from build123d import *

# Parameters (mm, degrees)
BOSS_EXTRUDE2_DEPTH = 230
SKETCH2_R           = 3
CUT_EXTRUDE1_DEPTH  = 4
SKETCH3_R           = 1.55
CUT_EXTRUDE2_DEPTH  = 4
LPATTERN1_COUNT     = 12
LPATTERN1_PITCH     = 20
SKETCH4_W           = 103
SKETCH4_H           = 312
SKETCH4_R           = 11.05
SKETCH4_R_2         = 1.55
SKETCH4_W_2         = 10
SKETCH4_H_2         = 12
BOSS_EXTRUDE3_DEPTH = 4.75
SKETCH5_R           = 1.25
CUT_EXTRUDE3_DEPTH  = 10


with BuildPart() as part:
    # Sketch1 → Boss-Extrude2 (new body)
    with BuildSketch(Plane.XY):
        Polygon((0.5, 2), (0.5, 0), (8.5, 0), (8.5, 2), (9, 2), (9, 5.5), (0, 5.5), (0, 2), align=None)
    extrude(amount=BOSS_EXTRUDE2_DEPTH)

    # Sketch2 → Cut-Extrude1 (cut)
    with BuildSketch(Plane(origin=(0, 0, 0), x_dir=(-1, 0, 0), z_dir=(0, -1, 0))):
        with Locations(Location((-4.5, -225, 0), (0, 0, 90))):
            Circle(SKETCH2_R)
    cut_extrude1 = extrude(amount=-CUT_EXTRUDE1_DEPTH, mode=Mode.SUBTRACT)

    # Sketch3 → Cut-Extrude2 (cut)
    with BuildSketch(Plane(origin=(0, 4, 0), x_dir=(-1, 0, 0), z_dir=(0, -1, 0))):
        with Locations(Location((-4.5, -225, 0), (0, 0, 90))):
            Circle(SKETCH3_R)
    cut_extrude2 = extrude(amount=-CUT_EXTRUDE2_DEPTH, mode=Mode.SUBTRACT)

    # LPattern1: Cut-Extrude1, Cut-Extrude2 ×12
    with Locations(*[(0, 0, -i * LPATTERN1_PITCH) for i in range(1, LPATTERN1_COUNT)]):
        add(cut_extrude1, mode=Mode.SUBTRACT)
        add(cut_extrude2, mode=Mode.SUBTRACT)

    # Sketch4 → Boss-Extrude3 (add)
    with BuildSketch(Plane(origin=(0, 5.5, 0), x_dir=(1, 0, 0), z_dir=(0, 1, 0))):
        with Locations((16.5, -126)):
            Rectangle(SKETCH4_W, SKETCH4_H)
        with Locations(Location((20, -235, 0), (0, 0, 270))):
            Circle(SKETCH4_R, mode=Mode.SUBTRACT)
        with Locations(Location((20, 6, 0), (0, 0, 270))):
            Circle(SKETCH4_R_2, mode=Mode.SUBTRACT)
        with Locations(Location((4.5, -225, 0), (0, 0, 90))):
            Circle(SKETCH4_R_2, mode=Mode.SUBTRACT)
        with Locations(Location((4.5, -205, 0), (0, 0, 90))):
            Circle(SKETCH4_R_2, mode=Mode.SUBTRACT)
        with Locations(Location((4.5, -185, 0), (0, 0, 90))):
            Circle(SKETCH4_R_2, mode=Mode.SUBTRACT)
        with Locations(Location((4.5, -165, 0), (0, 0, 90))):
            Circle(SKETCH4_R_2, mode=Mode.SUBTRACT)
        with Locations(Location((4.5, -145, 0), (0, 0, 90))):
            Circle(SKETCH4_R_2, mode=Mode.SUBTRACT)
        with Locations(Location((4.5, -125, 0), (0, 0, 90))):
            Circle(SKETCH4_R_2, mode=Mode.SUBTRACT)
        with Locations(Location((4.5, -105, 0), (0, 0, 90))):
            Circle(SKETCH4_R_2, mode=Mode.SUBTRACT)
        with Locations(Location((4.5, -85, 0), (0, 0, 90))):
            Circle(SKETCH4_R_2, mode=Mode.SUBTRACT)
        with Locations(Location((4.5, -65, 0), (0, 0, 90))):
            Circle(SKETCH4_R_2, mode=Mode.SUBTRACT)
        with Locations(Location((4.5, -45, 0), (0, 0, 90))):
            Circle(SKETCH4_R_2, mode=Mode.SUBTRACT)
        with Locations(Location((4.5, -25, 0), (0, 0, 90))):
            Circle(SKETCH4_R_2, mode=Mode.SUBTRACT)
        with Locations(Location((4.5, -5, 0), (0, 0, 90))):
            Circle(SKETCH4_R_2, mode=Mode.SUBTRACT)
        with Locations((20, 17)):
            Rectangle(SKETCH4_W_2, SKETCH4_H_2, mode=Mode.SUBTRACT)
    extrude(amount=BOSS_EXTRUDE3_DEPTH)

    # Sketch5 → Cut-Extrude3 (cut)
    with BuildSketch(Plane(origin=(0, 10.25, 0), x_dir=(1, 0, 0), z_dir=(0, 1, 0))):
        with Locations(Location((35.5, -250.5, 0), (0, 0, 270))):
            Circle(SKETCH5_R)
        with Locations(Location((4.5, -250.5, 0), (0, 0, 270))):
            Circle(SKETCH5_R)
        with Locations(Location((35.5, -219.5, 0), (0, 0, 270))):
            Circle(SKETCH5_R)
    extrude(amount=-CUT_EXTRUDE3_DEPTH, mode=Mode.SUBTRACT)


solid = part.part
Model file for the job. Use its own axes, mm. A direction names the side the tool comes from. Give positions to 0.01 mm unless a question says otherwise; leave off trailing zeros. Loops run counter-clockwise (first coordinate to the right, second up) from the corner with the lowest first, then second, coordinate; pieces in that order, holes last.
1) Flat gauge pins, fed straight in: pin 1 Ø3.5 at (x, z) = (4.5, 105) entering from +Y; pin 2 Ø3 at (x, y) = (5, 2) entering from -Z; pin 3 Ø4 at (y, z) = (3, 132.5) entering from +X; pin 4 Ø2.5 at (x, z) = (4.5, 205) entering from -Y. Where does each tip first touch, or does it go through?
2) Saw through at A-A (z = 235). Write the cut outline in (x, y).
3) Pull direction Z, two halves, no side cores. Call faces 3 (the flat face through (3, 4, 4)), 4 (the flat face through (4, 3, 230)), 5 (the flat face through (4, 3, 0)): +Z half, -Z half, draft (parallel to the pull), parting line (faces both ways), or undercut.
4) Wall check: line 1 (X direction, y = 6.95, z = 250.5); line 2 (X direction, y = 8.5, z = 226); line 3 (X direction, y = 6, z = 25). Give the ranges that are in metal, low to high.
5) Tool access for faces 1 (the flat face through (3, 4, 144)), 2 (the flat face through (16, 10.25, 124)): list every direction of +Z, -Z, +X, -X, +Y, -Y with a clear straight run to the whole face (end or side of a thin tool).
Answer block:
1. pin 1: stops at y = 10.25
1. pin 2: stops at z = 0
1. pin 3: stops at x = 9
1. pin 4: passes through
2. outline: (-35, 5.5) - (8.95, 5.5) - (8.95, 10.25) - (-35, 10.25) - close; (31.05, 5.5) - (68, 5.5) - (68, 10.25) - (31.05, 10.25) - close
3. face 3: undercut
3. face 4: +Z half
3. face 5: -Z half
4. line 1: x = -35 to 3.25, 5.75 to 34.25, 36.75 to 68
4. line 2: x = -35 to 3.32, 5.68 to 13.59, 26.41 to 68
4. line 3: x = -35 to 2.95, 6.05 to 68
5. face 1: -Y
5. face 2: +Z, -Z, +X, -X, +Y
